The drawing under review shows one solid part. Ordinate dimensions are in mm from its lowest x, y, z. A direction names the side the tool comes from. Give positions to 0.01 mm unless a question says otherwise; leave off trailing zeros. Loops run counter-clockwise (first coordinate to the right, second up) from the corner with the lowest first, then second, coordinate; pieces in that order, holes last. Notation, with made-up numbers: (61, -6) - (65, -6) arc R17 cw to (65, 6) - close; hole circle Ø7 at (24, 63). An arc over 180 degrees is marked (long way). Answer as CSV lines item,"result".
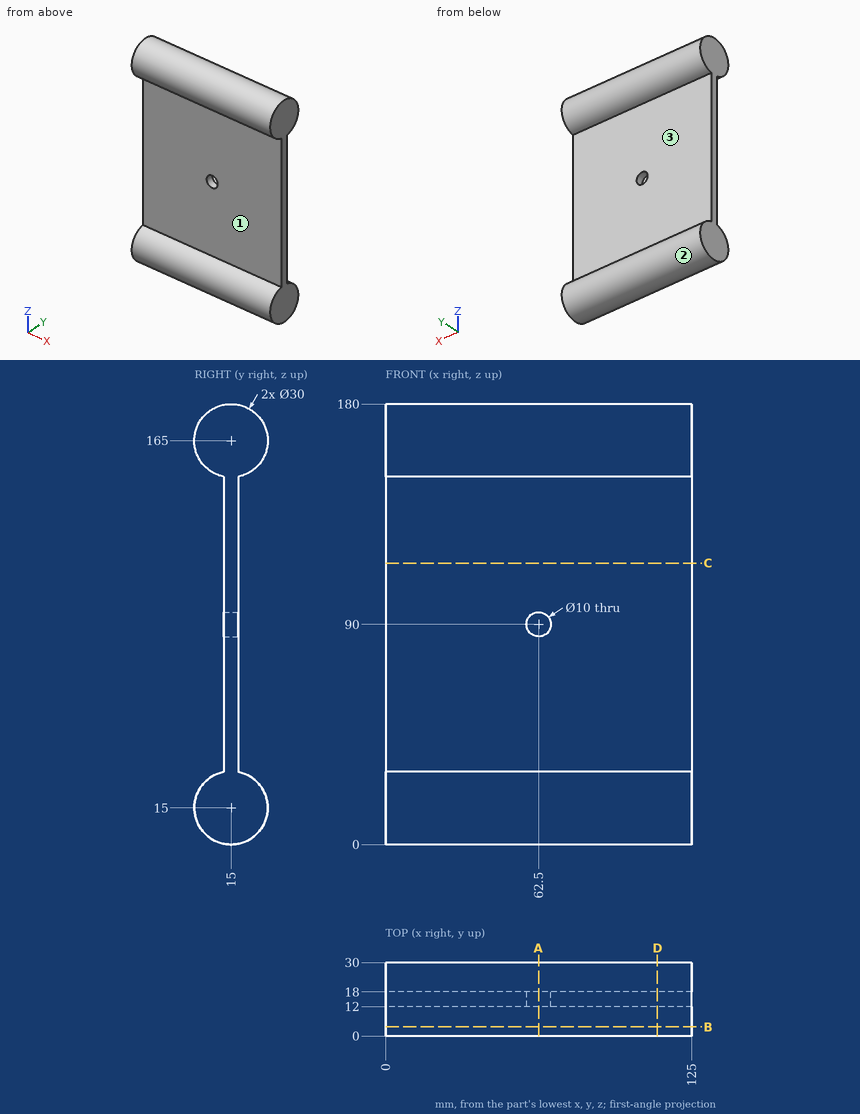
1) Consider section A-A on x = 62.5. Write out the cut boundary in (y, z).
From the geometry:
outline,"(12, 29.7) arc R15 ccw (long way) to (18, 29.7) - (18, 85) - (12, 85) - close; (12, 95) - (18, 95) - (18, 150.3) arc R15 ccw (long way) to (12, 150.3) - close"
2) Insertion check: P1, Ø4, axis at x = 111, y = 22.5, coming from the -Z side; P2, Ø8, axis at x = 87, z = 105, coming from the -Y side; P3, Ø6, axis at x = 82, y = 5.5, coming from the +Z side. Each pin has a flat end and moves straight along its axis. Give the tip position at first contact, or say it passes through.
From the geometry:
P1,"stops at z = 1.04"
P2,"stops at y = 12"
P3,"stops at z = 178.52"
3) Consider section B-B on y = 3.75. Write out the cut boundary in (x, z), and give its area (3 significant figures).
From the geometry:
outline,"(0, 5.08) - (125, 5.08) - (125, 24.92) - (0, 24.92) - close; (0, 155.08) - (125, 155.08) - (125, 174.92) - (0, 174.92) - close"
area,"4,960 mm^2"
4) Consider section D-D on x = 111. Write out the cut boundary in (y, z), and give its area (3 significant figures).
From the geometry:
outline,"(12, 29.7) arc R15 ccw (long way) to (18, 29.7) - (18, 150.3) arc R15 ccw (long way) to (12, 150.3) - close"
area,"2,130 mm^2"
5) Machinability: for the marked faces 1, 2 and 3, which of the approach directions +Z, -Z, +X, -X, +Y, -Y give a long, thin tool a straight path to every point of the face, cutting with its end or side? Answer none if there is none.
From the geometry:
face 1,"+X, -X, -Y"
face 2,"+X, -X"
face 3,"+X, -X, +Y"
6) Consider section C-C on z = 115. Write out the cut boundary in (x, y).
From the geometry:
outline,"(0, 12) - (125, 12) - (125, 18) - (0, 18) - close"
7) Wall thickness on line 1 (Z direction, x = 62.5, y = 14.5); line 2 (Y direction, x = 20.5, z = 131.5); line 3 (X direction, y = 17, z = 91.5): over which ranges is each line inside the solid? List them lowest first. Write a range as from..to.
From the geometry:
line 1,"z = 0.01..85, 95..179.99"
line 2,"y = 12..18"
line 3,"x = 0..57.73, 67.27..125"
